The drawing under review shows one solid part. Ordinate dimensions are in mm from its lowest x, y, z. A direction names the side the tool comes from. Round coordinates to 2 decimals unless told otherwise and drop trailing zeros. Write each loop counter-clockwise with the first axis right and the second up, starting at its lowest first coordinate (ties: lowest second). Pieces come first, ordered by that corner, then holes. Notation, with made-up numbers: (4, -28.5) -> (35, -28.5) arc R26 cw to (35, -1.5) -> close; hole circle Ø9 at (-5.5, 89.5). An arc over 180 degrees is marked (long way). Write item = value, one per line. Start each with the question number.
Item 1: For pin 1 Ø1.3 at (x, z) = (25, 26) entering from +Y; pin 2 Ø0.9 at (y, z) = (2, 17) entering from -X; pin 3 Ø12 at (x, z) = (24.5, 18.5) entering from -Y, all flat-tipped, find the tip position at first contact; note any pin that passes through.
Item 2: Mouldability with a two-part tool opening along X and no side actions: class the marked faces 3, 4 and 5 as released by +X, released by -X, zero draft, split by the parting line, or undercut.
Item 3: To check wall thickness, follow L1, parallel to Z at x = 25, y = 18.5; L2, parallel to Y at x = 34, z = 34.5. State the ranges of each line that lie inside material, in increasing order.
Item 4: Machinability: for the marked faces 1 and 2, which of the approach directions +Z, -Z, +X, -X, +Y, -Y give a long, thin tool a straight path to every point of the face, cutting with its end or side? Answer none if there is none.
Item 5: Add section B-B, the plane x = 25. State the section outline as (y, z) points, then the cut area to 3 significant figures.
Item 6: Add section A-A, the plane x = 5. State the section outline as (y, z) points, then the cut area to 3 significant figures.
Item 7: Add section C-C, the plane y = 29. State the section outline as (x, z) points, then the cut area to 3 significant figures.
Item 8: Add section D-D, the plane z = 12. State the section outline as (x, y) points, then the cut area to 3 significant figures.
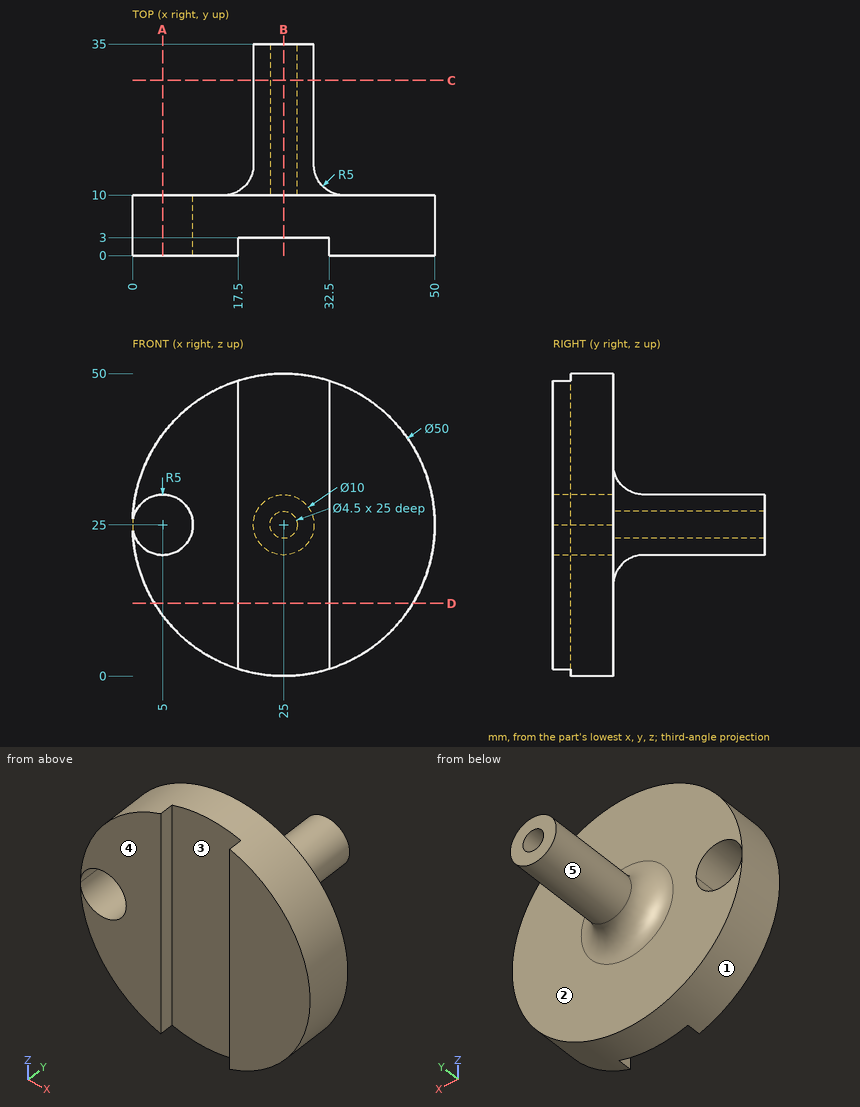
Result set:
q1.pin_1 = 10
q1.pin_2 = 1.17
q1.pin_3 = 3
q2.face_3 = undercut
q2.face_4 = zero draft
q2.face_5 = split by the parting line
q3.L1 = 20 to 22.75, 27.25 to 30
q3.L2 = 0 to 10
q4.face_1 = +Y, -Y
q4.face_2 = +Y
q5.outline = (3, 0) -> (10, 0) -> (10, 15) arc R5 cw to (15, 20) -> (35, 20) -> (35, 22.75) -> (10, 22.75) -> (10, 27.25) -> (35, 27.25) -> (35, 30) -> (15, 30) arc R5 cw to (10, 35) -> (10, 50) -> (3, 50) -> close
q5.area = 498 mm²
q6.outline = (0, 10) -> (10, 10) -> (10, 20) -> (0, 20) -> close; (0, 30) -> (10, 30) -> (10, 40) -> (0, 40) -> close
q6.area = 200 mm²
q7.outline = circle Ø10 at (25, 25); hole circle Ø4.5 at (25, 25)
q7.area = 62.6 mm²
q8.outline = (3.65, 0) -> (17.5, 0) -> (17.5, 3) -> (32.5, 3) -> (32.5, 0) -> (46.35, 0) -> (46.35, 10) -> (3.65, 10) -> close
q8.area = 382 mm²
